from build123d import *

# Parameters (mm, degrees)
ESQUISSE5_R        = 1.25
R_VOLUTION1_ANGLE  = 90
ESQUISSE6_R        = 1.25
BOSS_EXTRU_3_DEPTH = 1
ESQUISSE7_R        = 1.25
BOSS_EXTRU_4_DEPTH = 3


with BuildPart() as part:
    # Esquisse5 → Révolution1 (revolve)
    with BuildSketch(Plane.XY):
        with Locations((0, -3)):
            Circle(ESQUISSE5_R)
    revolve(axis=Axis((-1.070799248, 0, 0), (1, 0, 0)), revolution_arc=R_VOLUTION1_ANGLE)

    # Esquisse6 → Boss.-Extru.3 (add)
    with BuildSketch(Plane.XY):
        with Locations(Location((0, -3, 0), (0, 0, 270))):
            Circle(ESQUISSE6_R)
    extrude(amount=BOSS_EXTRU_3_DEPTH)

    # Esquisse7 → Boss.-Extru.4 (add)
    with BuildSketch(Plane(origin=(0, 0, 0), x_dir=(1, 0, 0), z_dir=(0, 1, 0))):
        with Locations(Location((0, 3, 0), (0, 0, 90))):
            Circle(ESQUISSE7_R)
    extrude(amount=BOSS_EXTRU_4_DEPTH)


solid = part.part
The model under review builds one solid part; all positions refer to its coordinate system, in mm. A direction names the side the tool comes from. Round coordinates to 2 decimals unless told otherwise and drop trailing zeros. Loops run counter-clockwise (first coordinate to the right, second up) from the corner with the lowest first, then second, coordinate; pieces in that order, holes last. Notation, with made-up numbers: M -19.5,-4.5 L 35.5,-4.5 A20 ccw 35.5,8.5 Z; hole C -20,43.5 d7. An arc over 180 degrees is marked long. Answer as a JSON object with one key per item and string values.
Item 1: We need section C-C, the plane x = 0.75. State the section outline as (y, z) points, and give its area (3 significant figures).
Check sheet entries:
{"outline": "M -4,0 A4 ccw 0,-4 L 3,-4 L 3,-2 L 0,-2 A2 cw -2,0 L -2,1 L -4,1 Z", "area": "17.4 mm2"}
Item 2: For line 1 along X through (y, z) = (-3.25, 0.5); line 2 along Y through (x, z) = (-0.65, 0.7); line 3 along Y through (x, z) = (-0.1, -1.45), list the stretches that pass through material, from the lowest coordinate up.
Check sheet entries:
{"line 1": "-1.22 to 1.22", "line 2": "-4.07 to -1.93", "line 3": "-3.99 to -0.99"}
Item 3: We need section A-A, the plane x = 0. State the section outline as (y, z) points.
Check sheet entries:
{"outline": "M -4.25,0 A4.25 ccw 0,-4.25 L 3,-4.25 L 3,-1.75 L 0,-1.75 A1.75 cw -1.75,0 L -1.75,1 L -4.25,1 Z"}
Item 4: Clearance check with a flat-ended pin moving along its axis: P1, Ø3, axis at y = -3.5, z = -3.5, coming from the +X side. State where the tip first meets the part, or that it passes through.
Check sheet entries:
{"P1": "x = 1.17"}
Item 5: Tool access review of faces 1 (the face through (0.38, -4.19, 0.49)), 2 (the face through (-0.38, 1.48, -4.19)), 3 (the face through (0, -3, 1)): name each direction out of +Z, -Z, +X, -X, +Y, -Y from which nothing blocks a thin tool from reaching the whole face with its end or side.
Check sheet entries:
{"face 1": "+Z", "face 2": "+Y", "face 3": "+Z, +X, -X, +Y, -Y"}
Item 6: We need section B-B, the plane z = 0.4. State the section outline as (x, y) points, and give its area (3 significant figures).
Check sheet entries:
{"outline": "C 0,-3 d2.5", "area": "4.91 mm2"}
